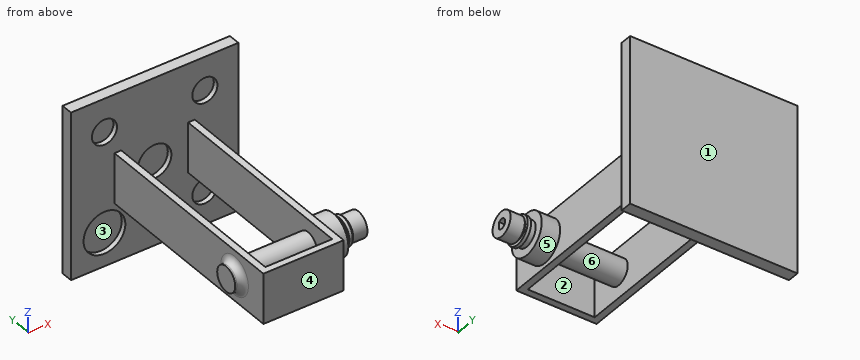
Autodesk Inventor part; units mm, degrees
ref_plane "Work Plane1" through (38.5, 20, 0) normal (1, 0, 0) x (0, 0, -1)
ref_plane "YZ Plane" through (0, 0, 0) normal (1, 0, 0) x (0, 1, 0)
ref_plane "XZ Plane" through (0, 0, 0) normal (0, 1, 0) x (-1, 0, 0)
sketch "Sketch1" plane through (0, 0, 0) normal (0, 1, 0) x (-1, 0, 0)
  line L0 (0, 0) -> (20, 0)
  line L1 (24, 15) -> (20, 15)
  line L2 (20, 15) -> (20, -15)
  line L3 (20, -15) -> (24, -15)
  line L4 (24, -15) -> (24, 15)
  line L5 (0, 0) -> (0, -10) construction
  line L6 (-24, 15) -> (-20, 15)
  line L7 (-20, 15) -> (-20, -15)
  line L8 (-20, -15) -> (-24, -15)
  line L9 (-24, -15) -> (-24, 15)
  point P0 (-20, 0)
  dimension "d0" = 20
  dimension "d1" = 30
  dimension "d2" = 4
  dimension "d3" = 15
extrude "Extrusion1" add sketch "Sketch1" along normal blind 120
sketch "Sketch2" plane through (-24, 0, -15) normal (-1, 0, 0) x (0, 0, 1)
  circle A0 centre (15, 20) radius 7.5
  line L0 (0, 0) -> (30, 0)
  point P0 (15, 0)
  dimension "d6" = 20
  dimension "d7" = 15
extrude "Extrusion2" cut sketch "Sketch2" against normal up to surface (48 mm away)
sketch "Sketch3" plane through (0, 0, 0) normal (0, -1, 0) x (1, 0, 0)
  line L0 (24, 15) -> (24, -15)
  line L1 (-24, -15) -> (-24, 15)
  line L2 (24, -15) -> (-24, -15)
  line L3 (20, 15) -> (24, 15)
  line L4 (-24, 15) -> (24, 15)
  point P0 (0, 0)
extrude "Extrusion3" add sketch "Sketch3" along normal blind 4
sketch "Sketch4" plane through (24, 120, 15) normal (1, 0, 0) x (0, 0, -1)
  circle A0 centre (15, -100) radius 7.5
  circle A1 centre (15, -100) radius 12.5
  point P0 (15, -120)
  dimension "d12" = 25
extrude "Extrusion4" cut sketch "Sketch4" against normal blind 1
sketch "Sketch6" plane through (0, 120, 0) normal (0, 1, 0) x (1, 0, 0)
  line L0 (-50, -50) -> (50, -50)
  line L1 (50, -50) -> (50, 50)
  line L2 (50, 50) -> (-50, 50)
  line L3 (-50, 50) -> (-50, -50)
  line L4 (-50, -50) -> (50, 50) construction
  line L5 (50, -50) -> (-50, 50) construction
  circle A0 centre (-30, 30) radius 12.5
  circle A1 centre (-30, -30) radius 7.5
  circle A2 centre (30, 30) radius 7.5
  circle A3 centre (30, -30) radius 7.5
  circle A4 centre (0, 0) radius 10
  dimension "d15" = 100
  dimension "d16" = 100
  dimension "d17" = 30
  dimension "d18" = 25
  dimension "d20" = 15
  dimension "d21" = 20
extrude "Extrusion5" add sketch "Sketch6" along normal blind 3
sketch "Sketch7" plane through (0, 123, 0) normal (0, 1, 0) x (1, 0, 0)
  line L0 (50, 50) -> (-50, 50)
  line L1 (-50, 50) -> (-50, -50)
  line L2 (-50, -50) -> (50, -50)
  line L3 (50, -50) -> (50, 50)
  circle A0 centre (-30, 30) radius 12.5
  circle A1 centre (-30, -30) radius 7.5
  circle A2 centre (30, 30) radius 7.5
  circle A3 centre (30, -30) radius 7.5
  circle A4 centre (0, 0) radius 10
extrude "Extrusion6" add sketch "Sketch7" along normal blind 4 contours L3 L2 L1 L0 | A0 | A1 | A2 | A3 | A4
sketch "Sketch8" plane through (24, -4, 15) normal (1, 0, 0) x (0, 0, -1)
  circle A0 centre (15, 24) radius 12.5
  circle A1 centre (15, 24) radius 7.5
  point P0 (15, 4)
extrude "Extrusion7" add sketch "Sketch8" along normal blind 11 and the other way blind 1
sketch "Sketch9" plane through (-24, -4, -15) normal (-1, 0, 0) x (0, 0, 1)
  circle A0 centre (15, 24) radius 7.5
  point P0 (15, 4)
extrude "Extrusion8" add sketch "Sketch9" along normal blind 5 and the other way blind 74
sketch "Sketch10" plane through (50, 20, 0) normal (1, 0, 0) x (0, 0, -1)
  circle A0 centre (0, 0) radius 7.5
  circle A1 centre (0, 0) radius 3
  line L0 (2.2361, -2) -> (-2.2361, -2)
  point P0 (0, -20)
  dimension "d34" = 6
  dimension "d35" = 2
extrude "Extrusion9" cut sketch "Sketch10" against normal blind 10 contours A1 L0 picked at (0.8351, -0.0457)
ref_plane "Work Plane1" through (38.5, 20, 0) normal (1, 0, 0) x (0, 0, -1)
sketch "Sketch11" plane through (38.5, 20, 0) normal (1, 0, 0) x (0, 0, -1)
  circle A0 centre (0, 0) radius 7.5
  circle A1 centre (0, 0) radius 6
  point P0 (0, -20)
  dimension "d39" = 12
extrude "Extrusion10" cut sketch "Sketch11" along normal blind 3
sketch "Sketch12" plane through (38.5, 20, 0) normal (1, 0, 0) x (0, 0, -1)
  circle A0 centre (0, 0) radius 7.5
  circle A1 centre (0, 0) radius 7.5
  circle A2 centre (0, 0) radius 7.5
  circle A3 centre (0, 0) radius 6.5
  circle A4 centre (0, 0) radius 8.5
  point P0 (0, -20)
  dimension "d42" = 13
  dimension "d43" = 17
extrude "Extrusion11" add sketch "Sketch12" along normal blind 2 contours A0 | A4
fillet "Fillet1" radius 4 1 edges at (-24, 20, -7.5)
equation "\"d3\" = 0.5 * d1"
properties part number "manufacturing link-4" material "Steel, Mild"
Geometry check sheet. Reference: the model listing, model coordinates, mm. Face numbers are marked on the shaded views. A direction names the side the tool comes from. Round coordinates to 2 decimals unless told otherwise and drop trailing zeros. Loops run counter-clockwise (first coordinate to the right, second up) from the corner with the lowest first, then second, coordinate; pieces in that order, holes last. Notation, with made-up numbers: (80.25, -10) - (121.25, -10) arc R20 ccw to (121.25, 28) - close; hole circle Ø11 at (34, 59). An arc over 180 degrees is marked (long way). Write item = value, one per line. Start each with the question number.
1. Depth check by flat-ended pin: pin 1 (15 mm diameter, centred on y = 46, z = 1.5, fed in from -X); pin 2 (12 mm diameter, centred on y = 17, z = 2, fed in from -X); pin 3 (5 mm diameter, centred on y = 49.5, z = -2, fed in from +X); pin 4 (10 mm diameter, centred on x = 12.5, y = 63, fed in from +Z). Enter the tip coordinate at first touch or a pass-through.
2. Section check C-C on x = 30. Enter the section's corners in (y, z), then the cut area to 3 significant figures.
3. Section check A-A on x = 0. Enter the section's corners in (y, z), then the cut area to 3 significant figures.
4. Section check D-D on z = -30. Enter the section's corners in (x, y).
5. Thickness scan on line 1 (X direction, y = 120.8, z = -30); line 2 (Z direction, x = 30, y = 121). Record the ranges inside material, lowest first.
6. Section check B-B on y = 51. Enter the section's corners in (x, z), then the cut area to 3 significant figures.
7. Set-up check for the marked faces 4, 5 and 6: record each of +Z, -Z, +X, -X, +Y, -Y from which the full face is reachable in a straight line by a thin tool's end or side.
8. Mould release check, pull along Y, two halves, no side actions. Record for the marked faces 1, 2 and 3: released by +Y, released by -Y, zero draft, split by the parting line, or undercut.
Working result:
q1.pin_1 = -24
q1.pin_2 = -29
q1.pin_3 = 24
q1.pin_4 = through
q2.outline = circle Ø25 at (20, 0); (120, -50) - (127, -50) - (127, 50) - (120, 50) - (120, 37.5) - (123, 37.5) - (123, 22.5) - (120, 22.5) - (120, -22.5) - (123, -22.5) - (123, -37.5) - (120, -37.5) - close
q2.area = 1,100 mm^2
q3.outline = (-4, -15) - (0, -15) - (0, 15) - (-4, 15) - close; circle Ø15 at (20, 0); (120, -50) - (127, -50) - (127, 50) - (120, 50) - (120, 10) - (123, 10) - (123, -10) - (120, -10) - close
q3.area = 937 mm^2
q4.outline = (-50, 120) - (-42.5, 120) - (-42.5, 123) - (-17.5, 123) - (-17.5, 120) - (22.5, 120) - (22.5, 123) - (37.5, 123) - (37.5, 120) - (50, 120) - (50, 127) - (-50, 127) - close
q5.line_1 = -50 to -42.5, -17.5 to 22.5, 37.5 to 50
q5.line_2 = -50 to -37.5, -22.5 to 22.5, 37.5 to 50
q6.outline = (-24, -15) - (-20, -15) - (-20, 15) - (-24, 15) - close; (20, -15) - (24, -15) - (24, 15) - (20, 15) - close
q6.area = 240 mm^2
q7.face_4 = +Z, -Z, +X, -X, -Y
q7.face_5 = +X
q7.face_6 = none
q8.face_1 = released by +Y
q8.face_2 = undercut
q8.face_3 = released by -Y
